Design review of the part built by this model. Coordinates are the model's own, in mm. A direction names the side the tool comes from. Coordinates: 2 decimals unless noted, no trailing zeros. Loops run counter-clockwise (first coordinate to the right, second up) from the corner with the lowest first, then second, coordinate; pieces in that order, holes last. Notation, with made-up numbers: (-14, -14) -> (-3, -14) arc R19 ccw to (-3, -1) -> close; hole circle Ø6 at (10, -25). An arc over 180 degrees is marked (long way). Answer in a Markdown table with one row per item.
```python
from build123d import *

# Parameters (mm, degrees)
SKETCH1_R           = 2.1
BOSS_EXTRUDE1_DEPTH = 65
FILLET1_R           = 1.5


with BuildPart() as part:
    # Sketch1 → Boss-Extrude1 (new body)
    with BuildSketch(Plane(origin=(0, 0, 0), x_dir=(1, 0, 0), z_dir=(0, 1, 0))):
        Polygon((0, 0), (7, 0), (7, 1.5), (3.56901309, 1.5), (3.56901309, 2.5), (7.26901309, 6.2), (12.73098691, 6.2), (16.43098691, 2.5), (16.43098691, 1.5), (13, 1.5), (13, 0), (20.018554527, 0), (20.018554527, 6.993482935), (18.518554527, 6.993482935), (18.518554527, 3.562496025), (17.518554527, 3.562496025), (13.777987766, 7.26901309), (13.777987766, 12.73098691), (17.518554527, 16.447701982), (18.518554527, 16.447701982), (18.518554527, 13.45318801), (20.018554527, 13.45318801), (20.018554527, 20), (13, 20), (13, 18.5), (16.43098691, 18.5), (16.43098691, 17.5), (12.73098691, 13.795754461), (7.26901309, 13.795754461), (3.56901309, 17.5), (3.56901309, 18.5), (7, 18.5), (7, 20), (0, 20), (0, 13.45318801), (1.5, 13.45318801), (1.5, 16.447701982), (2.5, 16.447701982), (6.209487856, 12.733957701), (6.209487856, 7.271983881), (2.5, 3.562496025), (1.5, 3.562496025), (1.5, 6.993482935), (0, 6.993482935), align=None)
        with Locations(Location((10, 10, 0), (0, 0, 270))):
            Circle(SKETCH1_R, mode=Mode.SUBTRACT)
    extrude(amount=BOSS_EXTRUDE1_DEPTH)

    # Fillet1
    fillet1_edges = [part.edges().sort_by_distance(p)[0] for p in [
        (0, 32.5, -20),
        (20.018554527, 32.5, -20),
        (20.018554527, 32.5, 0),
        (0, 32.5, 0),
    ]]
    fillet(fillet1_edges, radius=FILLET1_R)


solid = part.part
```
(1) For pin 1 (2.5 mm diameter, centred on y = 18, z = -10, fed in from +X); pin 2 (1.6 mm diameter, centred on x = 11, y = 24.5, fed in from +Z); pin 3 (0.8 mm diameter, centred on y = 42, z = -19.5, fed in from +X), all flat-tipped, find the tip position at first contact; note any pin that passes through.
Evaluation:
| item | result |
|---|---|
| pin 1 | stops at x = 13.78 |
| pin 2 | stops at z = -6.2 |
| pin 3 | stops at x = 19.89 |
(2) Draft analysis for pull direction Z (two halves, no side actions). For faces 4 (the flat face through (10, 32, -13.796)), 5 (the flat face through (19, 32, -6.993)), 6 (the flat face through (16, 32, 0)), 7 (the flat face through (15, 32, -1.5)), state which applies: pulls with the +Z half, pulls with the -Z half, needs draft (parallel to the pull), parting line crosses it, or undercut.
Evaluation:
| item | result |
|---|---|
| face 4 | pulls with the -Z half |
| face 5 | undercut |
| face 6 | pulls with the +Z half |
| face 7 | undercut |
(3) Tool access review of faces 1 (the flat face through (18.519, 32, -5)), 2 (the flat face through (13.778, 32, -10)), 3 (the flat face through (10, 32, -6.2)): name each direction out of +Z, -Z, +X, -X, +Y, -Y from which nothing blocks a thin tool from reaching the whole face with its end or side.
Evaluation:
| item | result |
|---|---|
| face 1 | +Y, -Y |
| face 2 | +X, +Y, -Y |
| face 3 | +Z, +Y, -Y |
(4) Take a section at C-C on x = 10. Give the boundary of the cut face in (y, z), and give its area (3 significant figures).
Evaluation:
| item | result |
|---|---|
| outline | (0, -13.8) -> (65, -13.8) -> (65, -12.1) -> (0, -12.1) -> close; (0, -7.9) -> (65, -7.9) -> (65, -6.2) -> (0, -6.2) -> close |
| area | 221 mm² |
(5) Take a section at A-A on z = -10. Give the boundary of the cut face in (x, y), and give its area (3 significant figures).
Evaluation:
| item | result |
|---|---|
| outline | (6.21, 0) -> (7.9, 0) -> (7.9, 65) -> (6.21, 65) -> close; (12.1, 0) -> (13.78, 0) -> (13.78, 65) -> (12.1, 65) -> close |
| area | 219 mm² |
(6) To check wall thickness, follow probe 1 along Z at (x, y) = (14.5, 61); probe 2 along X at (y, z) = (34, -15.25); probe 3 along X at (y, z) = (38, -10). State the ranges of each line that lie inside material, in increasing order.
Evaluation:
| item | result |
|---|---|
| probe 1 | z = -20 to -18.5, -15.57 to -13.45, -6.55 to -4.43, -1.5 to 0 |
| probe 2 | x = 0 to 1.5, 3.7 to 5.82, 14.18 to 16.31, 18.52 to 20.02 |
| probe 3 | x = 6.21 to 7.9, 12.1 to 13.78 |
(7) Take a section at B-B on x = 4.5. Give the boundary of the cut face in (y, z), and give its area (3 significant figures).
Evaluation:
| item | result |
|---|---|
| outline | (0, -20) -> (65, -20) -> (65, -18.5) -> (0, -18.5) -> close; (0, -16.57) -> (65, -16.57) -> (65, -14.45) -> (0, -14.45) -> close; (0, -5.56) -> (65, -5.56) -> (65, -3.43) -> (0, -3.43) -> close; (0, -1.5) -> (65, -1.5) -> (65, 0) -> (0, 0) -> close |
| area | 472 mm² |
(8) Take a section at D-D on z = -15. Give the boundary of the cut face in (x, y), and give its area (3 significant figures).
Evaluation:
| item | result |
|---|---|
| outline | (0, 0) -> (1.5, 0) -> (1.5, 65) -> (0, 65) -> close; (3.95, 0) -> (6.07, 0) -> (6.07, 65) -> (3.95, 65) -> close; (13.93, 0) -> (16.06, 0) -> (16.06, 65) -> (13.93, 65) -> close; (18.52, 0) -> (20.02, 0) -> (20.02, 65) -> (18.52, 65) -> close |
| area | 471 mm² |
